```python
from build123d import *

# Parameters (mm, degrees)
F0_W     = 10.5
F0_H     = 13
F0_W_2   = 2.7
F0_H_2   = 1.54
F1_DEPTH = 0.7
F2_DEPTH = 1.85
F3_W     = 1.9751354622
F3_H     = 1.54
F3_W_2   = 2.0054427082
F4_DEPTH = 1
F3_W_3   = 1.6171073075
F3_H_2   = 0.5545145935
F3_H_3   = 2.2898169597
F3_H_4   = 0.6118393503
F5_DEPTH = 1.6


with BuildPart() as f1:
    # F0 (on Top) → F1 (new body)
    with BuildSketch(Plane.XY):
        Rectangle(F0_W, F0_H)
        with Locations((-3.0680515347, -1.0410206797)):
            Rectangle(F0_W_2, F0_H_2, mode=Mode.SUBTRACT)
        with Locations((-0.0680515347, -1.0410206797)):
            Rectangle(F0_W_2, F0_H_2, mode=Mode.SUBTRACT)
        with Locations((2.9319484653, -1.0410206797)):
            Rectangle(F0_W_2, F0_H_2, mode=Mode.SUBTRACT)
        with Locations((-3.0306075118, 2.78879628)):
            Rectangle(F0_W_2, F0_H_2, mode=Mode.SUBTRACT)
        with Locations((-0.0306075118, 2.78879628)):
            Rectangle(F0_W_2, F0_H_2, mode=Mode.SUBTRACT)
        with Locations((2.9693924882, 2.78879628)):
            Rectangle(F0_W_2, F0_H_2, mode=Mode.SUBTRACT)
        with Locations((-3.0680515347, -1.0410206797)):
            Rectangle(F0_W_2, F0_H_2)
        with Locations((-3.0306075118, 2.78879628)):
            Rectangle(F0_W_2, F0_H_2)
        with Locations((-0.0306075118, 2.78879628)):
            Rectangle(F0_W_2, F0_H_2)
        with Locations((-0.0680515347, -1.0410206797)):
            Rectangle(F0_W_2, F0_H_2)
        with Locations((2.9319484653, -1.0410206797)):
            Rectangle(F0_W_2, F0_H_2)
        with Locations((2.9693924882, 2.78879628)):
            Rectangle(F0_W_2, F0_H_2)
    extrude(amount=F1_DEPTH)

    # F0 (on Top) → F2 (join)
    with BuildSketch(Plane.XY):
        with Locations((-3.0680515347, -1.0410206797)):
            Rectangle(F0_W_2, F0_H_2)
        with Locations((-0.0680515347, -1.0410206797)):
            Rectangle(F0_W_2, F0_H_2)
        with Locations((2.9319484653, -1.0410206797)):
            Rectangle(F0_W_2, F0_H_2)
        with Locations((2.9693924882, 2.78879628)):
            Rectangle(F0_W_2, F0_H_2)
        with Locations((-0.0306075118, 2.78879628)):
            Rectangle(F0_W_2, F0_H_2)
        with Locations((-3.0306075118, 2.78879628)):
            Rectangle(F0_W_2, F0_H_2)
    extrude(amount=F2_DEPTH)

    # F3 (on face) → F4 (join)
    with BuildSketch(Plane.XY):
        Polygon((-3.7234942429, -1.8110206797), (-3.7234942429, -4.0597501211), (0.5570839276, -4.0597501211), (0.5570839276, -1.8110206797), (-1.4180515347, -1.8110206797), (-1.4180515347, -0.2710206797), (0.5570839276, -0.2710206797), (0.5570839276, 0), (-3.7234942429, 0), (-3.7234942429, -0.2710206797), (-1.7180515347, -0.2710206797), (-1.7180515347, -1.8110206797), align=None)
        with Locations((-0.4304838036, -1.0410206797)):
            Rectangle(F3_W, F3_H)
        with Locations((-2.7207728888, -1.0410206797)):
            Rectangle(F3_W_2, F3_H)
    extrude(amount=-F4_DEPTH)

    # F3 (on face) → F5 (join)
    with BuildSketch(Plane.XY):
        with Locations((2.9827450635, -0.5482779764)):
            Rectangle(F3_W_3, F3_H_2)
        with Locations((2.9827450635, 0.8738878002)):
            Rectangle(F3_W_3, F3_H_3)
        with Locations((2.9827450635, 2.3247159552)):
            Rectangle(F3_W_3, F3_H_4)
    extrude(amount=-F5_DEPTH)


solid = f1.part
```
Geometry check sheet. Reference: the model listing, model coordinates, mm. A direction names the side the tool comes from. Coordinates: 2 decimals unless noted, no trailing zeros. Order: outer loops, then holes, each group sorted by start corner. A loop starts at its lowest first (then second) coordinate and runs counter-clockwise, first axis right, second up.
Q1. Tool access check on faces 1 (the face through (-2, -2, -1)), 2 (the face through (-1.418, -1, 1)), 3 (the face through (0.557, -2.1, -0.5)), 4 (the face through (3.791, 1, -1)). Record the directions out of +Z, -Z, +X, -X, +Y, -Y that give a thin tool (end or side, any length) a straight path to the whole face; none if there is none.
Reply:
face 1: -Z, -X, +Y, -Y
face 2: +Z, +Y, -Y
face 3: -Z, +Y, -Y
face 4: -Z, +X, +Y, -Y
Q2. Sectioned sample at C-C on x = 0. Record the cut outline in (y, z).
Reply:
outline: (-6.5, 0) - (-4.06, 0) - (-4.06, -1) - (0, -1) - (0, 0) - (6.5, 0) - (6.5, 0.7) - (3.56, 0.7) - (3.56, 1.85) - (2.02, 1.85) - (2.02, 0.7) - (-0.27, 0.7) - (-0.27, 1.85) - (-1.81, 1.85) - (-1.81, 0.7) - (-6.5, 0.7) - close
Q3. Sectioned sample at B-B on y = -0.5. Record the cut outline in (x, z).
Reply:
outline: (-5.25, 0) - (-3.72, 0) - (-3.72, -1) - (0.56, -1) - (0.56, 0) - (2.17, 0) - (2.17, -1.6) - (3.79, -1.6) - (3.79, 0) - (5.25, 0) - (5.25, 0.7) - (4.28, 0.7) - (4.28, 1.85) - (1.58, 1.85) - (1.58, 0.7) - (1.28, 0.7) - (1.28, 1.85) - (-1.42, 1.85) - (-1.42, 0.7) - (-1.72, 0.7) - (-1.72, 1.85) - (-4.42, 1.85) - (-4.42, 0.7) - (-5.25, 0.7) - close
Q4. Sectioned sample at A-A on z = 1. Record the cut outline in (x, y), and give its area (3 significant figures).
Reply:
outline: (-4.42, -1.81) - (-1.72, -1.81) - (-1.72, -0.27) - (-4.42, -0.27) - close; (-4.38, 2.02) - (-1.68, 2.02) - (-1.68, 3.56) - (-4.38, 3.56) - close; (-1.42, -1.81) - (1.28, -1.81) - (1.28, -0.27) - (-1.42, -0.27) - close; (-1.38, 2.02) - (1.32, 2.02) - (1.32, 3.56) - (-1.38, 3.56) - close; (1.58, -1.81) - (4.28, -1.81) - (4.28, -0.27) - (1.58, -0.27) - close; (1.62, 2.02) - (4.32, 2.02) - (4.32, 3.56) - (1.62, 3.56) - close
area: 24.9 mm2
Q5. Draft check along X on faces 5 (the face through (-1.681, 3, 1)), 6 (the face through (-4.418, -1, 1)), 7 (the face through (1.619, 3, 1)), 8 (the face through (0, -1.811, 1)). Enter one of: released by +X, released by -X, zero draft, split by the parting line, or undercut.
Reply:
face 5: undercut
face 6: released by -X
face 7: undercut
face 8: zero draft
Q6. Sectioned sample at D-D on z = -0.75. Record the cut outline in (x, y).
Reply:
outline: (-3.72, -4.06) - (0.56, -4.06) - (0.56, 0) - (-3.72, 0) - close; (2.17, -0.83) - (3.79, -0.83) - (3.79, 2.63) - (2.17, 2.63) - close
Q7. Thickness scan on probe 1 along Y at (x, z) = (-2.75, 1.4); probe 2 along Z at (x, y) = (3.5, -2); probe 3 along Y at (x, z) = (-2.5, -0.75). Record the ranges inside material, lowest first.
Reply:
probe 1: y = -1.81 to -0.27, 2.02 to 3.56
probe 2: z = 0 to 0.7
probe 3: y = -4.06 to 0
Q8. Depth check by flat-ended pin: pin 1 Ø0.8 at (y, z) = (1.5, -1) entering from +X; pin 2 Ø0.6 at (x, z) = (-3.5, 1.5) entering from +Y; pin 3 Ø0.9 at (y, z) = (2.5, 1.5) entering from +X. Enter the tip coordinate at first touch or a pass-through.
Reply:
pin 1: stops at x = 3.79
pin 2: stops at y = 3.56
pin 3: stops at x = 4.32
